Input: part model. Units: mm. Frame: model coordinates. A direction names the side the tool comes from. Round coordinates to 2 decimals unless told otherwise and drop trailing zeros. Order: outer loops, then holes, each group sorted by start corner. A loop starts at its lowest first (then second) coordinate and runs counter-clockwise, first axis right, second up. Notation, with made-up numbers: (74.25, 29) -> (132.25, 29) arc R25 ccw to (132.25, 53) -> close; hole circle Ø4 at (-10, 68.5). An arc over 180 degrees is marked (long way). Use a Markdown table: item, result.
from build123d import *

# Parameters (mm, degrees)
PAD_DEPTH    = 20
SKETCH001_W  = 10
SKETCH001_H  = 2
PAD001_DEPTH = 3
SKETCH002_R  = 1.375
PAD002_DEPTH = 1.4
FILLET_R     = 0.7


with BuildPart() as part:
    # Sketch → Pad (new body)
    with BuildSketch(Plane.XY):
        with BuildLine():
            Line((-10.3, 0), (10.3, 0))
            ThreePointArc((10.3, 0), (10.794975, 0.205025), (11, 0.7))
            Line((11, 5.3), (11, 0.7))
            ThreePointArc((11, 5.3), (10.794975, 5.794975), (10.3, 6))
            Line((-5.914335, 6), (10.3, 6))
            ThreePointArc((-5.914335, 6), (-6.323047, 5.868291), (-6.577955, 5.522727))
            ThreePointArc((-9.5, 6), (-8.241799, 4.519617), (-6.577955, 5.522727))
            Line((-9.5, 6), (-9.5, 10.396598))
            ThreePointArc((-8.704163, 11.090006), (-9.259845, 10.924369), (-9.5, 10.396598))
            Line((-8.704163, 11.090006), (2.8, 9.5))
            ThreePointArc((2.8, 9.5), (4.196693, 9.355621), (5.6, 9.307419))
            Line((5.6, 9.307419), (8.2, 9.307419))
            ThreePointArc((8.2, 9.307419), (9.758568, 9.725036), (10.899519, 10.865987))
            ThreePointArc((10.899519, 10.865987), (10.625, 11.890506), (9.600482, 11.615987))
            ThreePointArc((8.2, 10.807418), (9.008569, 11.024074), (9.600482, 11.615987))
            Line((5.6, 10.807418), (8.2, 10.807418))
            ThreePointArc((3.003702, 10.986104), (4.29878, 10.852143), (5.6, 10.807418))
            Line((-9.452691, 12.693515), (3.003702, 10.986104))
            ThreePointArc((-9.452691, 12.693515), (-9.500111, 12.698377), (-9.547752, 12.7))
            Line((-10.3, 12.7), (-9.547752, 12.7))
            ThreePointArc((-10.3, 12.7), (-10.794975, 12.494975), (-11, 12))
            Line((-11, 6), (-11, 12))
            Line((-11, 0.7), (-11, 6))
            ThreePointArc((-11, 0.7), (-10.794975, 0.205025), (-10.3, 0))
        make_face()
    extrude(amount=PAD_DEPTH)

    # Sketch001 (on DatumPlane) → Pad001 (join)
    with BuildSketch(Plane.XZ.offset(-6)):
        with Locations((2, 19)):
            Rectangle(SKETCH001_W, SKETCH001_H)
    extrude(amount=-PAD001_DEPTH)

    # Sketch002 → Pad002 (join)
    with BuildSketch(Plane.XY):
        with Locations((6, 2.375)):
            Circle(SKETCH002_R)
        with Locations((-6, 2.375)):
            Circle(SKETCH002_R)
    extrude(amount=-PAD002_DEPTH)

    # Fillet
    fillet_edges = [part.edges().sort_by_distance(p)[0] for p in [
        (-3, 9, 19),
        (-3, 6, 19),
        (7, 9, 19),
        (7, 6, 19),
    ]]
    fillet(fillet_edges, radius=FILLET_R)


solid = part.part
1) Draft query along X for faces 1 (the face through (0, 0, 10)), 2 (the face through (-8.271, 4.525, 9.86)), 3 (the face through (4.281, 10.853, 9.86)), 4 (the face through (-11, 6, 10)). Return one class per face: released by +X, released by -X, zero draft, split by the parting line, or undercut.
Answer key:
| item | result |
|---|---|
| face 1 | zero draft |
| face 2 | undercut |
| face 3 | undercut |
| face 4 | released by -X |
2) Contact query for flat-ended pins moving along their axis: P1, Ø3, axis at x = -1, y = 5.5, coming from the -Z side; P2, Ø3, axis at x = 6.5, z = 13.5, coming from the +Y side; P3, Ø0.6, axis at x = 2.5, z = 19, coming from the +Y side. Output: stop coordinate, or through.
Answer key:
| item | result |
|---|---|
| P1 | stops at z = 0 |
| P2 | stops at y = 10.82 |
| P3 | stops at y = 11.1 |
3) Cut plane B-B on z = 7.5. Return loops of the section in (x, y).
Answer key:
| item | result |
|---|---|
| outline | (-11, 0.7) arc R0.7 ccw to (-10.3, 0) -> (10.3, 0) arc R0.7 ccw to (11, 0.7) -> (11, 5.3) arc R0.7 ccw to (10.3, 6) -> (-5.91, 6) arc R0.7 ccw to (-6.58, 5.52) arc R1.5 cw to (-9.5, 6) -> (-9.5, 10.4) arc R0.7 cw to (-8.7, 11.09) -> (2.8, 9.5) arc R20.45 ccw to (5.6, 9.31) -> (8.2, 9.31) arc R3.12 ccw to (10.9, 10.87) arc R0.75 ccw to (9.6, 11.62) arc R1.62 cw to (8.2, 10.81) -> (5.6, 10.81) arc R18.95 cw to (3, 10.99) -> (-9.45, 12.69) arc R0.7 ccw to (-9.55, 12.7) -> (-10.3, 12.7) arc R0.7 ccw to (-11, 12) -> close |
4) Set-up query: faces 5 (the face through (-4.73, 1.85, -0.69)), 6 (the face through (9.739, 9.714, 9.86)), 7 (the face through (-3, 10.3, 9.9)), 8 (the face through (7, 10.807, 10)). Return all of +Z, -Z, +X, -X, +Y, -Y with unobstructed straight access to the full face (end or side cutting, diameter ignored); none if empty.
Answer key:
| item | result |
|---|---|
| face 5 | -Z |
| face 6 | +Z, -Z, +X |
| face 7 | +Z, -Z |
| face 8 | +Z, -Z, +Y |
5) Cut plane A-A on x = 6. Return loops of the section in (y, z).
Answer key:
| item | result |
|---|---|
| outline | (0, 0) -> (1, 0) -> (1, -1.4) -> (3.75, -1.4) -> (3.75, 0) -> (6, 0) -> (6, 18) -> (9, 18) -> (9, 20) -> (0, 20) -> close; (9.31, 0) -> (10.81, 0) -> (10.81, 20) -> (9.31, 20) -> close |
6) Cut plane C-C on y = 3. Return loops of the section in (x, z), and give its area (3 significant figures).
Answer key:
| item | result |
|---|---|
| outline | (-11, 0) -> (-7.22, 0) -> (-7.22, -1.4) -> (-4.78, -1.4) -> (-4.78, 0) -> (4.78, 0) -> (4.78, -1.4) -> (7.22, -1.4) -> (7.22, 0) -> (11, 0) -> (11, 20) -> (-11, 20) -> close |
| area | 447 mm^2 |
7) Ray query, probe 1 along Y at (x, z) = (8, 0.25); probe 2 along Z at (x, y) = (7.5, 2.5); probe 3 along Y at (x, z) = (1.5, 9.5). Return the intervals inside material, ascending.
Answer key:
| item | result |
|---|---|
| probe 1 | y = 0 to 6, 9.31 to 10.81 |
| probe 2 | z = 0 to 20 |
| probe 3 | y = 0 to 6, 9.68 to 11.19 |
8) Cut plane D-D on x = 2. Return loops of the section in (y, z).
Answer key:
| item | result |
|---|---|
| outline | (0, 0) -> (6, 0) -> (6, 18) -> (9, 18) -> (9, 20) -> (0, 20) -> close; (9.61, 0) -> (11.12, 0) -> (11.12, 20) -> (9.61, 20) -> close |
